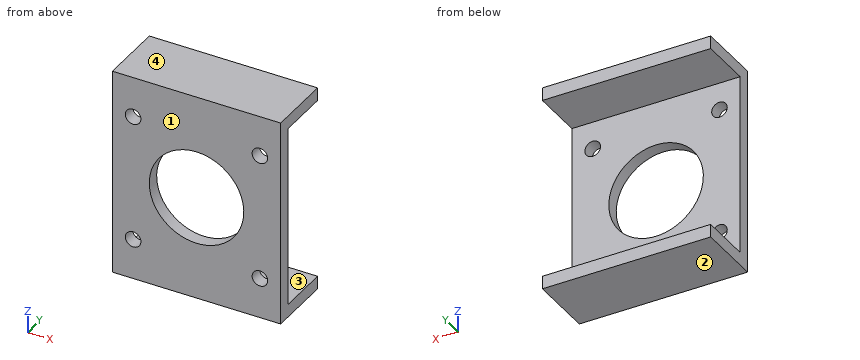
```python
from build123d import *

# Parameters (mm, degrees)
SKETCH1_W           = 41.148
SKETCH1_H           = 50.8
SKETCH1_R           = 11.557
SKETCH1_R_2         = 1.905
BOSS_EXTRUDE1_DEPTH = 3.175
SKETCH2_W           = 41.148
SKETCH2_H           = 3.175
BOSS_EXTRUDE2_DEPTH = 12.7


with BuildPart() as part:
    # Sketch1 → Boss-Extrude1 (new body)
    with BuildSketch(Plane(origin=(0, 0, 0), x_dir=(1, 0, 0), z_dir=(0, 1, 0))):
        Rectangle(SKETCH1_W, SKETCH1_H)
        with Locations(Location((0, 0, 0), (0, 0, 270))):
            Circle(SKETCH1_R, mode=Mode.SUBTRACT)
        with Locations(Location((-15.499999988, 15.499999988, 0), (0, 0, 270))):
            Circle(SKETCH1_R_2, mode=Mode.SUBTRACT)
        with Locations(Location((15.499999988, 15.499999988, 0), (0, 0, 270))):
            Circle(SKETCH1_R_2, mode=Mode.SUBTRACT)
        with Locations(Location((15.499999988, -15.499999988, 0), (0, 0, 270))):
            Circle(SKETCH1_R_2, mode=Mode.SUBTRACT)
        with Locations(Location((-15.499999988, -15.499999988, 0), (0, 0, 270))):
            Circle(SKETCH1_R_2, mode=Mode.SUBTRACT)
    extrude(amount=BOSS_EXTRUDE1_DEPTH)

    # Sketch2 → Boss-Extrude2 (add)
    with BuildSketch(Plane(origin=(0, 3.175, 0), x_dir=(1, 0, 0), z_dir=(0, 1, 0))):
        with Locations((0, -23.8125)):
            Rectangle(SKETCH2_W, SKETCH2_H)
        with Locations((0, 23.8125)):
            Rectangle(SKETCH2_W, SKETCH2_H)
    extrude(amount=BOSS_EXTRUDE2_DEPTH)


solid = part.part
```
Can you work these out from the model? Positions are in its coordinate system, mm. Face numbers are marked on the shaded views. Coordinates: 2 decimals unless noted, no trailing zeros. Loops run counter-clockwise (first coordinate to the right, second up) from the corner with the lowest first, then second, coordinate; pieces in that order, holes last. Notation, with made-up numbers: (51, 24.25) - (80, 24.25) arc R23 ccw to (80, 61.25) - close; hole circle Ø11 at (48.25, 38). An arc over 180 degrees is marked (long way). Use a Markdown table: item, result.
Item 1: We'd pull the mould along Z, two halves only. Please class the marked faces 1, 2, 3 and 4: released by +Z, released by -Z, zero draft, split by the parting line, or undercut.
Numbers:
| item | result |
|---|---|
| face 1 | zero draft |
| face 2 | released by -Z |
| face 3 | undercut |
| face 4 | released by +Z |
Item 2: I want a section at A-A on x = 15.5. Please give me the cut outline in (y, z) (3 decimals).
Numbers:
| item | result |
|---|---|
| outline | (0, -25.4) - (15.875, -25.4) - (15.875, -22.225) - (3.175, -22.225) - (3.175, -17.405) - (0, -17.405) - close; (0, -13.595) - (3.175, -13.595) - (3.175, 13.595) - (0, 13.595) - close; (0, 17.405) - (3.175, 17.405) - (3.175, 22.225) - (15.875, 22.225) - (15.875, 25.4) - (0, 25.4) - close |
Item 3: I want a section at D-D on x = 0. Please give me the cut outline in (y, z) (3 decimals).
Numbers:
| item | result |
|---|---|
| outline | (0, -25.4) - (15.875, -25.4) - (15.875, -22.225) - (3.175, -22.225) - (3.175, -11.557) - (0, -11.557) - close; (0, 11.557) - (3.175, 11.557) - (3.175, 22.225) - (15.875, 22.225) - (15.875, 25.4) - (0, 25.4) - close |
Item 4: Will these pins go through, and if not, where does the flat tip stop? pin 1 (1 mm diameter, centred on x = -15, z = 6.5, fed in from +Y) (3 decimals); pin 2 (10 mm diameter, centred on x = 2.5, z = -17.5, fed in from +Y) (3 decimals).
Numbers:
| item | result |
|---|---|
| pin 1 | stops at y = 3.175 |
| pin 2 | stops at y = 15.875 |
Item 5: If I drill on probe 1 along X at (y, z) = (0.9, -15.5) (3 decimals); probe 2 along Z at (x, y) = (15.5, 1.35) (3 decimals); probe 3 along X at (y, z) = (2.3, 0), over which ranges is the centre line in solid material (lowest first)? Write a range as from..to.
Numbers:
| item | result |
|---|---|
| probe 1 | x = -20.574..-17.405, -13.595..13.595, 17.405..20.574 |
| probe 2 | z = -25.4..-17.405, -13.595..13.595, 17.405..25.4 |
| probe 3 | x = -20.57..-11.56, 11.56..20.57 |
Item 6: I want a section at C-C on y = 14. Please give me the cut outline in (x, z) (3 decimals).
Numbers:
| item | result |
|---|---|
| outline | (-20.574, -25.4) - (20.574, -25.4) - (20.574, -22.225) - (-20.574, -22.225) - close; (-20.574, 22.225) - (20.574, 22.225) - (20.574, 25.4) - (-20.574, 25.4) - close |
Item 7: I want a section at B-B on z = 15.5. Please give me the cut outline in (x, y) (3 decimals).
Numbers:
| item | result |
|---|---|
| outline | (-20.574, 0) - (-17.405, 0) - (-17.405, 3.175) - (-20.574, 3.175) - close; (-13.595, 0) - (13.595, 0) - (13.595, 3.175) - (-13.595, 3.175) - close; (17.405, 0) - (20.574, 0) - (20.574, 3.175) - (17.405, 3.175) - close |
